Part model, mm, in its own coordinate system. A direction names the side the tool comes from. Round coordinates to 2 decimals unless told otherwise and drop trailing zeros. Loops run counter-clockwise (first coordinate to the right, second up) from the corner with the lowest first, then second, coordinate; pieces in that order, holes last. Notation, with made-up numbers: (70, 41) - (119, 41) arc R18 cw to (119, 54) - close; hole circle Ø8 at (64.5, -24). An arc over 180 degrees is marked (long way). Put each result on its own line as item: value.
Autodesk Inventor part; units mm, degrees
ref_plane "YZ Plane" through (0, 0, 0) normal (1, 0, 0) x (0, 1, 0)
ref_plane "XZ Plane" through (0, 0, 0) normal (0, 1, 0) x (-1, 0, 0)
ref_plane "XY Plane" through (0, 0, 0) normal (0, 0, 1) x (1, 0, 0)
sketch "Sketch1" plane through (0, 0, 0) normal (0, 1, 0) x (-1, 0, 0)
  line L0 (38.4325, -41.9578) -> (13.0325, -41.9578)
  line L1 (13.0325, -41.9578) -> (13.0325, 16.4622)
  line L2 (13.0325, 16.4622) -> (38.4325, 16.4622)
  line L3 (38.4325, 16.4622) -> (38.4325, -41.9578)
  line L4 (38.4325, -41.9578) -> (-9.6784, 6.153) construction
  line L5 (38.4325, -41.9578) -> (38.4325, -16.5578)
  line L6 (38.4325, -16.5578) -> (-19.9875, -16.5578)
  line L7 (-19.9875, -16.5578) -> (-19.9875, -41.9578)
  line L8 (-19.9875, -41.9578) -> (38.4325, -41.9578)
  point P0 (0, 0)
  point P1 (13.0325, -16.5578)
  dimension "d0" = 25.4
  dimension "d1" = 58.42
  dimension "d2" = 45
extrude "Extrusion1" add sketch "Sketch1" along normal blind 2.286
chamfer "Chamfer1" distance 2.54 angle 45 1 edges at (-13.0325, 1.143, 16.4622)
chamfer "Chamfer2" distance 2.54 angle 45 4 edges at (-38.4325, 1.143, 16.4622) (19.9875, 1.143, -16.5578) (19.9875, 1.143, -41.9578) (-38.4325, 1.143, -41.9578)
fillet "Fillet1" radius 3.175 1 edges at (-13.0325, 1.143, -16.5578)
sketch "Sketch2" plane through (0, 2.286, 0) normal (0, 1, 0) x (1, 0, 0)
  circle A0 centre (-25.8595, 29.3848) radius 2.0828
  line L0 (17.4475, 41.9578) -> (-35.8925, 41.9578)
  line L1 (19.9875, 19.0978) -> (19.9875, 39.4178)
  line L2 (-38.4325, 39.4178) -> (-38.4325, -13.9222)
  point P0 (0, 0)
  dimension "d12" = 12.573
  dimension "d14" = 4.1656
  dimension "d23" = 12.573
extrude "Extrusion2" cut sketch "Sketch2" against normal blind 2.286
pattern_linear "Rectangular Pattern1" count 5 spacing 12.7 along (0, 0, 1) of "Extrusion2"
pattern_linear "Rectangular Pattern2" count 5 spacing 12.7 along (1, 0, 0) of "Extrusion2"
properties part number "ShortenedVersaGusset 90o"
1. Two-plate mould, pull along Z, no slides. Class faces 3 (the cylindrical face through (-12.08, 1.16, -15.65)), 4 (the cylindrical face through (-26.13, 1.16, 6.65)), 5 (the flat face through (-10, 1, -41.958)), 6 (the cylindrical face through (-26.31, 1.16, -1.95)): pulls with the +Z half, pulls with the -Z half, needs draft (parallel to the pull), parting line crosses it, or undercut.
A:
face 3: pulls with the +Z half
face 4: undercut
face 5: pulls with the -Z half
face 6: undercut
2. Probe line 1 along X through (y, z) = (0.5, -29); line 2 along Z through (x, y) = (-27, 1.8); line 3 along X through (y, z) = (1.55, 6). List the from-to ranges inside material, lowest first. Write a range as [from, to].
A:
line 1: x = [-38.43, -27.91], [-23.81, -15.21], [-11.11, -2.51], [1.59, 10.19], [14.29, 19.99]
line 2: z = [-41.96, -31.13], [-27.64, -18.43], [-14.94, -5.73], [-2.24, 6.97], [10.46, 16.46]
line 3: x = [-38.43, -13.03]
3. Pin check, flat tips, straight feed: P1, Ø3.5, axis at x = -0.46, z = -29.38, coming from the +Y side; P2, Ø5, axis at x = -9.5, z = -31, coming from the -Y side; P3, Ø1.1, axis at x = 8, y = 1, coming from the +Z side. Stop position of each tip, or through.
A:
P1: passes through
P2: stops at y = 0
P3: stops at z = -16.56
4. Band-saw the part on D-D (z = -1). List the corners of the cut face in (x, y).
A:
outline: (-38.43, 0) - (-13.03, 0) - (-13.03, 2.29) - (-38.43, 2.29) - close
5. Tool access for faces 1 (the flat face through (4, 1, -16.558)), 2 (the cylindrical face through (0.66, 1.16, -31.14)): list every direction of +Z, -Z, +X, -X, +Y, -Y with a clear straight run to the whole face (end or side of a thin tool).
A:
face 1: +Z, +X, +Y, -Y
face 2: +Y, -Y
6. Band-saw the part on C-C (y = 1.3). Give the number of separate pieces and of enclosed holes in the cut face, plus the area to 3 significant figures.
A:
separate pieces: 1
enclosed holes: 7
area: 2,210 mm²
7. Band-saw the part on B-B (x = 13). List the corners of the cut face in (y, z).
A:
outline: (0, -41.96) - (2.29, -41.96) - (2.29, -31.32) - (0, -31.32) - close; (0, -27.45) - (2.29, -27.45) - (2.29, -16.56) - (0, -16.56) - close
8. Band-saw the part on A-A (x = -26). List the corners of the cut face in (y, z).
A:
outline: (0, -41.96) - (2.29, -41.96) - (2.29, -31.46) - (0, -31.46) - close; (0, -27.31) - (2.29, -27.31) - (2.29, -18.76) - (0, -18.76) - close; (0, -14.61) - (2.29, -14.61) - (2.29, -6.06) - (0, -6.06) - close; (0, -1.91) - (2.29, -1.91) - (2.29, 6.64) - (0, 6.64) - close; (0, 10.79) - (2.29, 10.79) - (2.29, 16.46) - (0, 16.46) - close
